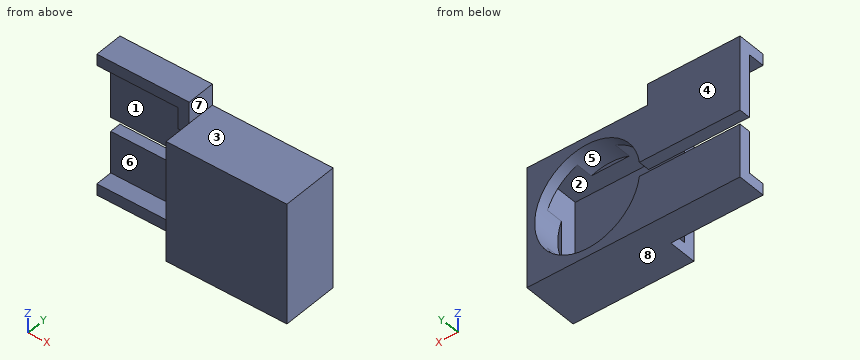
Autodesk Inventor part; units mm, degrees
ref_plane "YZ Plane" through (0, 0, 0) normal (1, 0, 0) x (0, 1, 0)
ref_plane "XZ Plane" through (0, 0, 0) normal (0, 1, 0) x (-1, 0, 0)
ref_plane "XY Plane" through (0, 0, 0) normal (0, 0, 1) x (1, 0, 0)
sketch "Sketch1" plane through (0, 0, 0) normal (0, 1, 0) x (-1, 0, 0)
  line L0 (-4.25, -4.25) -> (4.25, -4.25)
  line L1 (4.25, -4.25) -> (4.25, 4.25)
  line L2 (4.25, 4.25) -> (-4.25, 4.25)
  line L3 (-4.25, 4.25) -> (-4.25, -4.25)
  line L4 (-4.25, -4.25) -> (4.25, 4.25) construction
  line L5 (4.25, -4.25) -> (-4.25, 4.25) construction
  circle A0 centre (0, 0) radius 3.7
  line L6 (10.75, 0.5) -> (3.6661, 0.5)
  line L7 (10.75, -0.5) -> (3.6661, -0.5)
  line L8 (6.6744, 0) -> (-5, 0)
  line L9 (4.25, 4.25) -> (4.25, 5.75)
  line L10 (4.25, 5.75) -> (10.75, 5.75)
  line L11 (10.75, 5.75) -> (10.75, -4.25)
  line L12 (10.75, -4.25) -> (4.25, -4.25)
  point P0 (4.25, 0.5)
  point P1 (4.25, -0.5)
  dimension "d0" = 8.5
  dimension "d1" = 8.5
  dimension "d2" = 7.4
  dimension "d6" = 1
  dimension "d9" = 1.5
  dimension "d10" = 6.5
extrude "Extrusion1" add sketch "Sketch1" along normal mid plane 4
shell "Shell2" thickness 0.8 removed faces 1 at (-10.75, 0.6667, 2.4167)
extrude "Extrusion2" cut sketch "Sketch1" along normal up to next contours L7 A0 L8 L1 | L1 L6 L11 L7 | L8 A0 | A0 L8 | L8 A0 L6 L1
extrude "Extrusion3" cut sketch "Sketch1" against normal up to next contours L1 L7 L11 L12 | L1 L6 L11 L7 | L9 L10 L11 L6 L1
properties part number "camera"
Read the model definition and answer for the solid it produces. Units are mm, in the model's axes. Face numbers are marked on the shaded views. A direction names the side the tool comes from. Coordinates: 2 decimals unless noted, no trailing zeros. Loops run counter-clockwise (first coordinate to the right, second up) from the corner with the lowest first, then second, coordinate; pieces in that order, holes last. Notation, with made-up numbers: (51, -25.75) - (94, -25.75) arc R8 cw to (94, -13.75) - close; hole circle Ø5 at (42, 76.25). An arc over 180 degrees is marked (long way). Answer in a Markdown table with one row per item.
Q1. Find section D-D on z = 0. Write down the section's boundary in (x, y).
Here are the results:
| item | result |
|---|---|
| outline | (-4.25, -2) - (4.25, -2) - (4.25, 2) - (3.7, 2) - (3.7, 0) - (3.45, 0) - (3.45, -1.2) - (-4.25, -1.2) - close |
Q2. Straight lines are drawn through the part: line 1 along Z through (x, y) = (3.25, 1.1); line 2 along Z through (x, y) = (-4.5, 1.8); line 3 along Y through (x, z) = (-2.75, 3). For each, find the intervals that lie inside material, in ascending order. Write a range as [from, to].
Here are the results:
| item | result |
|---|---|
| line 1 | z = [-4.25, -3.45], [3.45, 4.25] |
| line 2 | z = [-4.25, -0.5], [0.5, 5.75] |
| line 3 | y = [-2, -1.2], [1.2, 2] |
Q3. Find section A-A on x = 0. Write down the section's boundary in (y, z).
Here are the results:
| item | result |
|---|---|
| outline | (-2, -4.25) - (2, -4.25) - (2, -3.7) - (0, -3.7) - (0, -3.45) - (-1.2, -3.45) - (-1.2, 3.45) - (0, 3.45) - (0, 3.7) - (2, 3.7) - (2, 4.25) - (-2, 4.25) - close |
Q4. Find section B-B on y = -0.3. Write down the section's boundary in (x, z).
Here are the results:
| item | result |
|---|---|
| outline | (-4.25, -4.25) - (4.25, -4.25) - (4.25, 4.25) - (-4.25, 4.25) - (-4.25, 3.45) - (3.45, 3.45) - (3.45, -3.45) - (-4.25, -3.45) - close |
Q5. Find section C-C on z = -2.25. Write down the section's boundary in (x, y), plus the area to 3 significant figures.
Here are the results:
| item | result |
|---|---|
| outline | (-10.75, 1.2) - (-2.94, 1.2) - (-2.94, 2) - (-10.75, 2) - close; (-4.25, -2) - (4.25, -2) - (4.25, 2) - (2.94, 2) - (2.94, 1.2) - (3.45, 1.2) - (3.45, -1.2) - (-4.25, -1.2) - close |
| area | 16.0 mm^2 |
Q6. For the marked faces 5, 6, 7 and 8, determine the directions among +Z, -Z, +X, -X, +Y, -Y from which every point of the face is accessible in a straight line to the end or side of a thin tool.
Here are the results:
| item | result |
|---|---|
| face 5 | +Y |
| face 6 | -X |
| face 7 | +Z, +X, +Y, -Y |
| face 8 | -Z, +X, -X, +Y, -Y |
Q7. Given P1, Ø2, axis at x = -0.5, z = 2, coming from the +Y side; P2, Ø1.6, axis at y = -1.5, z = -1.5, coming from the -X side; P3, Ø2.5, axis at x = -8.5, z = -1.5, coming from the -Y side, each flat-ended and moving along its own axis, determine where each tip first touches the part or whether it passes through.
Here are the results:
| item | result |
|---|---|
| P1 | stops at y = -1.2 |
| P2 | stops at x = -4.25 |
| P3 | stops at y = 1.2 |
Q8. The mould has two halves that part along Y. Classify the marked faces 1, 2, 3 and 4: pulls with the +Y half, pulls with the -Y half, needs draft (parallel to the pull), parting line crosses it, or undercut.
Here are the results:
| item | result |
|---|---|
| face 1 | undercut |
| face 2 | undercut |
| face 3 | needs draft |
| face 4 | pulls with the +Y half |
